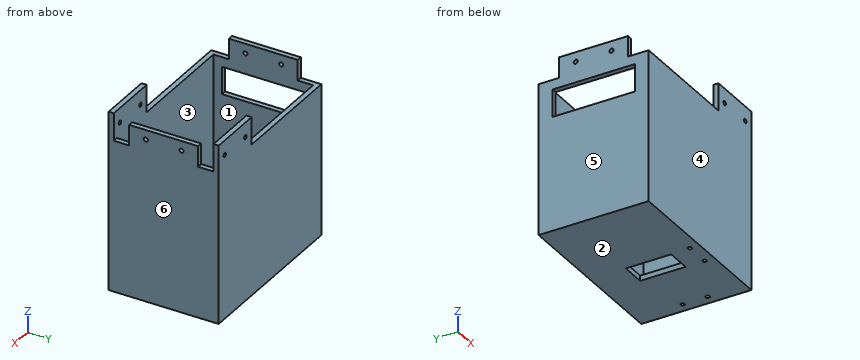
Autodesk Inventor part; units mm, degrees
ref_plane "Work Plane1" through (0, 40, 0) normal (0, 1, 0) x (-1, 0, 0)
ref_plane "Work Plane2" through (62.5, 0, 0) normal (1, 0, 0) x (0, 1, 0)
ref_plane "XY Plane" through (0, 0, 0) normal (0, 0, 1) x (1, 0, 0)
sketch "Sketch1" plane through (0, 0, 0) normal (0, 0, 1) x (1, 0, 0)
  line L0 (0, 0) -> (125, 0)
  line L1 (125, 0) -> (125, 80)
  line L2 (125, 80) -> (0, 80)
  line L3 (0, 80) -> (0, 0)
  dimension "d0" = 125
  dimension "d1" = 80
extrude "Extrusion1" add sketch "Sketch1" along normal blind 110
shell "Shell1" thickness 3.75 removed faces 1 at (83.3333, 26.6667, 110)
sketch "Sketch2" plane through (0, 0, 0) normal (0, 0, -1) x (-1, 0, 0)
  line L0 (0, 80) -> (0, 0)
  line L1 (-125, 80) -> (0, 80)
  line L2 (0, 0) -> (-125, 0)
  line L3 (-125, 0) -> (-125, 80)
  circle A0 centre (-118, 27.634) radius 1.5
  circle A1 centre (-118, 45.733) radius 1.5
  circle A2 centre (-79.9, 7) radius 1.5
  circle A3 centre (-61.929, 7) radius 1.5
  line L4 (-62.4, 53.8768) -> (-79.9, 53.8768)
  line L5 (-79.9, 53.8768) -> (-79.9, 20.8768)
  line L6 (-79.9, 20.8768) -> (-62.4, 20.8768)
  line L7 (-62.4, 20.8768) -> (-62.4, 53.8768)
  dimension "d22" = 3
  dimension "d23" = 3
  dimension "d24" = 7
  dimension "d25" = 7
  dimension "d26" = 27.634
  dimension "d46" = 45.733
  dimension "d77" = 3
  dimension "d78" = 3
  dimension "d79" = 7
  dimension "d80" = 7
  dimension "d81" = 45.1
  dimension "d82" = 63.071
  dimension "d83" = 45.1
  dimension "d84" = 20.8768
  dimension "d85" = 33
  dimension "d86" = 17.5
extrude "Extrusion6" cut sketch "Sketch2" against normal blind 20 contours A0 | A1 | A2 | A3 | L7 L6 L5 L4
sketch "Sketch6" plane through (0, 80, 0) normal (0, 1, 0) x (1, 0, 0)
  line L0 (0, -110) -> (125, -110)
  line L1 (125, -110) -> (85, -110)
  line L2 (85, -110) -> (85, -130)
  line L3 (85, -130) -> (125, -130)
  line L4 (125, -130) -> (125, -110)
  point P0 (0, 0)
  dimension "d53" = 40
  dimension "d54" = 20
extrude "Extrusion8" add sketch "Sketch6" against normal blind 3.75
ref_plane "Work Plane1" through (0, 40, 0) normal (0, 1, 0) x (-1, 0, 0)
mirror "Mirror1" about plane through (0, 40, 0) normal (0, 1, 0) of "Extrusion8"
sketch "Sketch7" plane through (0, 0, 0) normal (-1, 0, 0) x (0, 0, 1)
  line L0 (110, 3.75) -> (110, 76.25)
  line L1 (110, 15) -> (125, 15)
  line L2 (125, 15) -> (125, 65)
  line L3 (125, 65) -> (110, 65)
  line L4 (110, 65) -> (110, 15)
  line L5 (130, 76.25) -> (110, 76.25)
  line L6 (130, 3.75) -> (110, 3.75)
  point P0 (0, 0)
  dimension "d58" = 15
  dimension "d59" = 50
  dimension "d60" = 11.25
  dimension "d61" = 11.25
extrude "Extrusion9" add sketch "Sketch7" against normal blind 3.75
ref_plane "Work Plane2" through (62.5, 0, 0) normal (1, 0, 0) x (0, 1, 0)
mirror "Mirror2" about plane through (62.5, 0, 0) normal (1, 0, 0) of "Extrusion9"
sketch "Sketch8" plane through (0, 0, 0) normal (-1, 0, 0) x (0, 0, 1)
  line L0 (103, 70) -> (83, 70)
  line L1 (83, 70) -> (83, 10)
  line L2 (83, 10) -> (103, 10)
  line L3 (103, 10) -> (103, 70)
  line L4 (110, 3.75) -> (110, 15)
  line L5 (0, 0) -> (110, 0)
  line L6 (0, 80) -> (110, 80)
  dimension "d70" = 20
  dimension "d71" = 60
  dimension "d72" = 7
  dimension "d73" = 10
  dimension "d74" = 10
extrude "Extrusion11" cut sketch "Sketch8" against normal blind 10
sketch "Sketch9" plane through (0, 0, 0) normal (-1, 0, 0) x (0, 0, 1)
  circle A0 centre (118, 53) radius 1.5
  circle A1 centre (118, 27) radius 1.5
  line L0 (110, 15) -> (125, 15)
  line L1 (125, 15) -> (125, 65)
  line L2 (125, 65) -> (110, 65)
  point P0 (0, 0)
  dimension "d87" = 3
  dimension "d88" = 3
  dimension "d89" = 12
  dimension "d90" = 7
  dimension "d91" = 12
  dimension "d92" = 7
extrude "Extrusion12" cut sketch "Sketch9" against normal blind 200
sketch "Sketch10" plane through (0, 0, 0) normal (0, -1, 0) x (1, 0, 0)
  circle A0 centre (92.5, 119.3503) radius 1.5
  circle A1 centre (117.5, 119.3503) radius 1.5
  line L0 (125, 0) -> (125, 130)
  line L1 (85, 110) -> (85, 130)
  line L2 (85, 130) -> (125, 130)
  point P0 (0, 0)
  dimension "d95" = 3
  dimension "d96" = 3
  dimension "d97" = 7.5
  dimension "d98" = 7.5
  dimension "d99" = 10.6497
  dimension "d100" = 10.6497
extrude "Extrusion13" cut sketch "Sketch10" against normal blind 100
properties part number "Main Part"
The model under review builds one solid part; all positions refer to its coordinate system, in mm. Face numbers are marked on the shaded views. A direction names the side the tool comes from. Coordinates: 2 decimals unless noted, no trailing zeros. Loops run counter-clockwise (first coordinate to the right, second up) from the corner with the lowest first, then second, coordinate; pieces in that order, holes last. Notation, with made-up numbers: (-5.5, -33) -> (14.5, -33) arc R25 cw to (14.5, 0) -> close; hole circle Ø8 at (66, 0.5). An arc over 180 degrees is marked (long way). Use a Markdown table: item, result. Add a question column.
1. Add section A-A on y = 12.5. Write out the cut boundary in (x, z), plus the area to 3 significant figures.
2. Machinability: for the marked faces 1 and 2, which of the approach directions +Z, -Z, +X, -X, +Y, -Y give a long, thin tool a straight path to every point of the face, cutting with its end or side? Answer none if there is none.
3. Add section D-D on y = 72. Write out the cut boundary in (x, z).
4. Add section B-B on z = 60. Write out the cut boundary in (x, y).
5. Clearance check with flat-ended pins moving along their axes: pin 1 Ø1.1 at (x, y) = (122.5, 70.5) entering from +Z; pin 2 Ø1.8 at (x, z) = (117.5, 119.35) entering from -Y; pin 3 Ø3 at (y, z) = (2, 125) entering from -X; pin 4 Ø6 at (x, y) = (37, 54) entering from +Z. State where each tip first meets the part, or that it passes through.
6. Draft analysis for pull direction X (two halves, no side actions). For the marked faces 3, 4, 5 and 6, state which applies: pulls with the +X half, pulls with the -X half, needs draft (parallel to the pull), parting line crosses it, or undercut.
7. To check wall thickness, follow line 1 (X direction, y = 74.5, z = 13); line 2 (Z direction, x = 117.5, y = 2.2); line 3 (Y direction, x = 44, z = 84.5). State the ranges of each line that lie inside material, in increasing order.
8. Add section C-C on x = 110.5. Write out the cut boundary in (y, z), plus the area to 3 significant figures.
Returned:
| question | item | result |
|---|---|---|
| 1 | outline | (0, 0) -> (125, 0) -> (125, 110) -> (121.25, 110) -> (121.25, 3.75) -> (3.75, 3.75) -> (3.75, 83) -> (0, 83) -> close; (0, 103) -> (3.75, 103) -> (3.75, 110) -> (0, 110) -> close |
| 1 | area | 1,190 mm² |
| 2 | face 1 | +Z |
| 2 | face 2 | -Z, +X, -X, +Y, -Y |
| 3 | outline | (0, 0) -> (125, 0) -> (125, 110) -> (121.25, 110) -> (121.25, 3.75) -> (3.75, 3.75) -> (3.75, 110) -> (0, 110) -> close |
| 4 | outline | (0, 0) -> (125, 0) -> (125, 80) -> (0, 80) -> close; hole (3.75, 3.75) -> (121.25, 3.75) -> (121.25, 76.25) -> (3.75, 76.25) -> close |
| 5 | pin 1 | stops at z = 110 |
| 5 | pin 2 | passes through |
| 5 | pin 3 | stops at x = 85 |
| 5 | pin 4 | stops at z = 3.75 |
| 6 | face 3 | undercut |
| 6 | face 4 | needs draft |
| 6 | face 5 | pulls with the -X half |
| 6 | face 6 | pulls with the +X half |
| 7 | line 1 | x = 0 to 3.75, 121.25 to 125 |
| 7 | line 2 | z = 0 to 117.85, 120.85 to 130 |
| 7 | line 3 | y = 0 to 3.75, 76.25 to 80 |
| 8 | outline | (0, 0) -> (80, 0) -> (80, 130) -> (76.25, 130) -> (76.25, 3.75) -> (3.75, 3.75) -> (3.75, 130) -> (0, 130) -> close |
| 8 | area | 1,250 mm² |
